from build123d import *
from build123d.topology import SkipClean

# Parameters (mm, degrees)
BOSS_EXTRUDE1_DEPTH = 2
SKETCH2_R           = 3.75
BOSS_EXTRUDE2_DEPTH = 1
SKETCH3_R           = 2.75
CUT_EXTRUDE1_DEPTH  = 1


with BuildPart() as part:
    # Sketch1 → Boss-Extrude1 (new body)
    with BuildSketch(Plane(origin=(0, 0, 0), x_dir=(1, 0, 0), z_dir=(0, 1, 0))):
        with BuildLine():
            Line((0.5625, 3.707572487), (5.45, 2.96605799))
            ThreePointArc((5.45, 2.96605799), (8, 0), (5.45, -2.96605799))
            Line((5.45, -2.96605799), (0.5625, -3.707572487))
            ThreePointArc((0.5625, -3.707572487), (0, -3.75), (-0.5625, -3.707572487))
            Line((-0.5625, -3.707572487), (-5.45, -2.96605799))
            ThreePointArc((-5.45, -2.96605799), (-8, 0), (-5.45, 2.96605799))
            Line((-5.45, 2.96605799), (-0.5625, 3.707572487))
            ThreePointArc((-0.5625, 3.707572487), (0, 3.75), (0.5625, 3.707572487))
        make_face()
    extrude(amount=BOSS_EXTRUDE1_DEPTH)

    # Sketch2 → Boss-Extrude2 (add)
    with SkipClean():  # the faces are left unmerged after this step: merging them gives an invalid solid
        with BuildSketch(Plane(origin=(0, 2, 0), x_dir=(1, 0, 0), z_dir=(0, 1, 0))):
            with Locations(Location((0, 0, 0), (0, 0, 81.373073441))):
                Circle(SKETCH2_R)
        extrude(amount=BOSS_EXTRUDE2_DEPTH)
    add(part.part.scale(1), mode=Mode.REPLACE)  # the faces are merged on a copy

    # Sketch3 → Cut-Extrude1 (cut)
    with BuildSketch(Plane.XZ):
        with Locations(Location((0, 0, 0), (0, 0, 270))):
            Circle(SKETCH3_R)
    extrude(amount=-CUT_EXTRUDE1_DEPTH, mode=Mode.SUBTRACT)


solid = part.part
The model under review builds one solid part; all positions refer to its coordinate system, in mm. A direction names the side the tool comes from. Round coordinates to 2 decimals unless told otherwise and drop trailing zeros. Write each loop counter-clockwise with the first axis right and the second up, starting at its lowest first coordinate (ties: lowest second). Pieces come first, ordered by that corner, then holes. Notation, with made-up numbers: (63.5, 54) -> (96.5, 54) arc R27 ccw to (96.5, 87) -> close; hole circle Ø6 at (-28, -11.75). An arc over 180 degrees is marked (long way). Answer as a JSON object with one key per item and string values.
1. Clearance check with flat-ended pins moving along their axes: pin 1 (1 mm diameter, centred on x = 3, y = 1.5, fed in from +Z); pin 2 (1.6 mm diameter, centred on x = 0, z = 0, fed in from -Y); pin 3 (1 mm diameter, centred on x = -3.5, y = 1, fed in from +Z). State where each tip first meets the part, or that it passes through.
Results found:
{"pin 1": "stops at z = 3.41", "pin 2": "stops at y = 1", "pin 3": "stops at z = 3.34"}
2. The part is to be moulded in two halves that separate along Z. For faces 3 (the face through (8, 1, 0)), 4 (the face through (0, 3, 0)), 5 (the face through (0, 1, 0)), say which applies: pulls with the +Z half, pulls with the -Z half, needs draft (parallel to the pull), parting line crosses it, or undercut.
Results found:
{"face 3": "parting line crosses it", "face 4": "needs draft", "face 5": "undercut"}
3. We need section C-C on z = 0. State the section outline as (x, y) points.
Results found:
{"outline": "(-8, 0) -> (-2.75, 0) -> (-2.75, 1) -> (2.75, 1) -> (2.75, 0) -> (8, 0) -> (8, 2) -> (3.75, 2) -> (3.75, 3) -> (-3.75, 3) -> (-3.75, 2) -> (-8, 2) -> close"}
4. Machinability: for faces 1 (the face through (-2.685, 0.493, 0.596)), 2 (the face through (1.9, 0, 2.4)), which of the approach directions +Z, -Z, +X, -X, +Y, -Y give a long, thin tool a straight path to every point of the face, cutting with its end or side? Answer none if there is none.
Results found:
{"face 1": "-Y", "face 2": "+Z, -Z, +X, -X, -Y"}
5. We need section D-D on x = 0. State the section outline as (y, z) points.
Results found:
{"outline": "(0, -3.75) -> (3, -3.75) -> (3, 3.75) -> (0, 3.75) -> (0, 2.75) -> (1, 2.75) -> (1, -2.75) -> (0, -2.75) -> close"}
6. We need section B-B on y = 0.8. State the section outline as (x, z) points.
Results found:
{"outline": "(-5.45, -2.97) -> (-0.56, -3.71) arc R3.75 ccw to (0.56, -3.71) -> (5.45, -2.97) arc R3 ccw to (5.45, 2.97) -> (0.56, 3.71) arc R3.75 ccw to (-0.56, 3.71) -> (-5.45, 2.97) arc R3 ccw to start; hole circle Ø5.5 at (0, 0)"}
7. To check wall thickness, follow line 1 along X through (y, z) = (0.65, 0); line 2 along Y through (x, z) = (0, -2); line 3 along Y through (x, z) = (3, 3). State the ranges of each line that lie inside material, in increasing order.
Results found:
{"line 1": "x = -8 to -2.75, 2.75 to 8", "line 2": "y = 1 to 3", "line 3": "y = 0 to 2"}
8. We need section A-A on y = 1.7. State the section outline as (x, z) points.
Results found:
{"outline": "(-5.45, -2.97) -> (-0.56, -3.71) arc R3.75 ccw to (0.56, -3.71) -> (5.45, -2.97) arc R3 ccw to (5.45, 2.97) -> (0.56, 3.71) arc R3.75 ccw to (-0.56, 3.71) -> (-5.45, 2.97) arc R3 ccw to start"}
